Build history of the part. All positions in model axes, mm. Round coordinates to 2 decimals unless told otherwise and drop trailing zeros. Loops run counter-clockwise (first coordinate to the right, second up) from the corner with the lowest first, then second, coordinate; pieces in that order, holes last.
from build123d import *

# Parameters (mm, degrees)
SKETCH1_W           = 300
SKETCH1_H           = 279.908
BOSS_EXTRUDE1_DEPTH = 3.175
SKETCH2_W           = 17
SKETCH2_H           = 17
SKETCH2_W_2         = 20.066
SKETCH2_H_2         = 15
SKETCH2_W_3         = 43.942
SKETCH2_H_3         = 7.62
CUT_EXTRUDE1_DEPTH  = 3.175
SKETCH3_R           = 12.7
SKETCH3_R_2         = 19.685
SKETCH3_R_3         = 1.6
CUT_EXTRUDE2_DEPTH  = 3.175


with BuildPart() as part:
    # Sketch1 → Boss-Extrude1 (new body)
    with BuildSketch(Plane(origin=(0, 0, 0), x_dir=(1, 0, 0), z_dir=(0, 1, 0))):
        with Locations((150, 139.954)):
            Rectangle(SKETCH1_W, SKETCH1_H)
    extrude(amount=BOSS_EXTRUDE1_DEPTH)

    # Sketch2 → Cut-Extrude1 (cut)
    with BuildSketch(Plane(origin=(0, 3.175, 0), x_dir=(1, 0, 0), z_dir=(0, 1, 0))):
        Polygon((283, 27), (273, 17), (283, 17), align=None)
        Polygon((273, 17), (263, 17), (263, 0), (283, 0), (283, 17), align=None)
        with Locations((291.5, 8.5)):
            Rectangle(SKETCH2_W, SKETCH2_H)
        Polygon((283, 27), (283, 17), (300, 17), (300, 114.24), (283, 114.24), align=None)
        Polygon((273, 262.908), (283, 252.908), (283, 262.908), align=None)
        Polygon((283, 165.668), (300, 165.668), (300, 262.908), (283, 262.908), (283, 252.908), align=None)
        with Locations((291.5, 271.408)):
            Rectangle(SKETCH2_W, SKETCH2_H)
        Polygon((283, 279.908), (263, 279.908), (263, 262.908), (273, 262.908), (283, 262.908), align=None)
        Polygon((17, 17), (27, 17), (17, 27), align=None)
        Polygon((17, 0), (37, 0), (37, 17), (27, 17), (17, 17), align=None)
        with Locations((8.5, 8.5)):
            Rectangle(SKETCH2_W, SKETCH2_H)
        Polygon((17, 114.24), (0, 114.24), (0, 17), (17, 17), (17, 27), align=None)
        Polygon((27, 262.908), (17, 262.908), (17, 252.908), align=None)
        Polygon((37, 262.908), (37, 279.908), (17, 279.908), (17, 262.908), (27, 262.908), align=None)
        with Locations((8.5, 271.408)):
            Rectangle(SKETCH2_W, SKETCH2_H)
        Polygon((0, 262.908), (0, 165.668), (17, 165.668), (17, 252.908), (17, 262.908), align=None)
        with Locations((93.345, 272.408)):
            Rectangle(SKETCH2_W_2, SKETCH2_H_2)
        Polygon((115.316, 264.908), (103.378, 264.908), (83.312, 264.908), (71.374, 264.908), (71.374, 257.288), (115.316, 257.288), align=None)
        with Locations((206.655, 272.408)):
            Rectangle(SKETCH2_W_2, SKETCH2_H_2)
        with Locations((206.655, 261.098)):
            Rectangle(SKETCH2_W_3, SKETCH2_H_3)
    extrude(amount=-CUT_EXTRUDE1_DEPTH, mode=Mode.SUBTRACT)

    # Sketch3 → Cut-Extrude2 (cut)
    with BuildSketch(Plane(origin=(0, 3.175, 0), x_dir=(1, 0, 0), z_dir=(0, 1, 0))):
        with Locations(Location((150, 167.873621066, 0), (0, 0, 270))):
            Circle(SKETCH3_R)
        with BuildLine():
            ThreePointArc((150, 180.573621066), (137.3, 167.873621066), (150, 155.173621066))
            Line((150, 155.173621066), (150, 180.573621066))
        make_face()
        with BuildLine():
            Line((150, 180.573621066), (150, 155.173621066))
            ThreePointArc((150, 155.173621066), (158.980256121, 158.893364945), (162.7, 167.873621066))
            ThreePointArc((162.7, 167.873621066), (158.980256121, 176.853877188), (150, 180.573621066))
        make_face()
        with Locations(Location((150, 241.858, 0), (0, 0, 270))):
            Circle(SKETCH3_R_2)
        with Locations(Location((150, 80, 0), (0, 0, 270))):
            Circle(SKETCH3_R)
        with Locations(Location((7.5, 155.668, 0), (0, 0, 270))):
            Circle(SKETCH3_R_3)
        with Locations(Location((7.5, 124.24, 0), (0, 0, 90))):
            Circle(SKETCH3_R_3)
        with Locations(Location((47, 7.5, 0), (0, 0, 90))):
            Circle(SKETCH3_R_3)
        with Locations(Location((73.312, 7.5, 0), (0, 0, 90))):
            Circle(SKETCH3_R_3)
        with Locations(Location((113.378, 7.5, 0), (0, 0, 90))):
            Circle(SKETCH3_R_3)
        with Locations(Location((133.378, 7.5, 0), (0, 0, 90))):
            Circle(SKETCH3_R_3)
        with Locations(Location((166.622, 7.5, 0), (0, 0, 270))):
            Circle(SKETCH3_R_3)
        with Locations(Location((186.622, 7.5, 0), (0, 0, 270))):
            Circle(SKETCH3_R_3)
        with Locations(Location((226.688, 7.5, 0), (0, 0, 270))):
            Circle(SKETCH3_R_3)
        with Locations(Location((253, 7.5, 0), (0, 0, 270))):
            Circle(SKETCH3_R_3)
        with Locations(Location((47, 272.408, 0), (0, 0, 270))):
            Circle(SKETCH3_R_3)
        with Locations(Location((73.312, 272.408, 0), (0, 0, 270))):
            Circle(SKETCH3_R_3)
        with Locations(Location((113.378, 272.408, 0), (0, 0, 270))):
            Circle(SKETCH3_R_3)
        with Locations(Location((133.378, 272.408, 0), (0, 0, 270))):
            Circle(SKETCH3_R_3)
        with Locations(Location((166.622, 272.408, 0), (0, 0, 90))):
            Circle(SKETCH3_R_3)
        with Locations(Location((186.622, 272.408, 0), (0, 0, 90))):
            Circle(SKETCH3_R_3)
        with Locations(Location((226.688, 272.408, 0), (0, 0, 90))):
            Circle(SKETCH3_R_3)
        with Locations(Location((253, 272.408, 0), (0, 0, 90))):
            Circle(SKETCH3_R_3)
        with Locations(Location((292.5, 155.668, 0), (0, 0, 90))):
            Circle(SKETCH3_R_3)
        with Locations(Location((292.5, 124.24, 0), (0, 0, 270))):
            Circle(SKETCH3_R_3)
    extrude(amount=-CUT_EXTRUDE2_DEPTH, mode=Mode.SUBTRACT)


solid = part.part
(1) Probe line 1 (Z direction, x = 253, y = 2.5); line 2 (X direction, y = 1.4, z = -242); line 3 (X direction, y = 3.05, z = -192). List the from-to ranges inside material, lowest first.
Responses:
line 1: z = -279.91 to -274.01, -270.81 to -9.1, -5.9 to 0
line 2: x = 17 to 130.32, 169.68 to 283
line 3: x = 17 to 283
(2) Slice it at B-B on y = 2.6. Count the separate pieces of the cut face and the enclosed holes in it, plus the area to 3 significant figures.
Responses:
separate pieces: 1
enclosed holes: 23
area: 71,000 mm2
(3) Pin check, flat tips, straight feed: P1, Ø1, axis at y = 1.5, z = -275, coming from the -X side; P2, Ø1.6, axis at y = 1, z = -220.5, coming from the -X side. Stop position of each tip, or through.
Responses:
P1: stops at x = 37
P2: stops at x = 17
(4) Slice it at A-A on z = -110. List the corners of the cut face in (x, y) (3 decimals), plus the area to 3 significant figures.
Responses:
outline: (17, 0) - (283, 0) - (283, 3.175) - (17, 3.175) - close
area: 845 mm2
(5) Pull direction X, two halves, no side cores. Call faces 1 (the face through (277.93, 1.61, -257.98)), 2 (the face through (137.6, 1.61, -82.75)), 3 (the face through (22, 2, -22)), 4 (the face through (148, 3.175, -142)): +X half, -X half, draft (parallel to the pull), parting line (faces both ways), or undercut.
Responses:
face 1: +X half
face 2: undercut
face 3: -X half
face 4: draft
